from build123d import *

# Parameters (mm, degrees)
F1_DEPTH = 20


with BuildPart() as f1:
    # F0 (on Front) → F1 (new body)
    with BuildSketch(Plane.XZ):
        with BuildLine():
            ThreePointArc((6, -33), (4.404002, -27.946999), (0, -25))
            ThreePointArc((0, -25), (3.349365, -12.5), (0, 0))
            ThreePointArc((0, 0), (2.776172, 4.64825), (1.956342, 10))
            ThreePointArc((1.956342, 10), (-4.515013, 6.983663), (-6, 0))
            ThreePointArc((-6, 0), (-25.5, 3.94398), (-45, 0))
            ThreePointArc((-45, 0), (-47.052036, 6.711726), (-53.605872, 9.222772))
            ThreePointArc((-53.605872, 9.222772), (-53.826207, 4.173647), (-50.976141, 0))
            ThreePointArc((-50.976141, 0), (-54.905427, -13.454553), (-50.976141, -26.909107))
            ThreePointArc((-50.976141, -26.909107), (-54.301232, -29.687561), (-55.689886, -33.792153))
            ThreePointArc((-55.689886, -33.792153), (-49.556723, -34.118029), (-45, -30))
            ThreePointArc((-45, -30), (-25.5, -33.215544), (-6, -30))
            ThreePointArc((-6, -30), (-0.709551, -34.338204), (6, -33))
        make_face()
    extrude(amount=F1_DEPTH)


solid = f1.part
Geometry: final body of the model. Coordinates: model frame, mm. Give positions to 0.01 mm unless a question says otherwise; leave off trailing zeros. Loops run counter-clockwise (first coordinate to the right, second up) from the corner with the lowest first, then second, coordinate; pieces in that order, holes last. Notation, with made-up numbers: M 32,56.25 L 49,56.25 A14 cw 49,72.25 Z; hole C 64,-17.5 d9. An arc over 180 degrees is marked long. Put each result on its own line as item: value. Start each with the question number.
1) Ray query, line 1 along Z through (x, y) = (1.5, -18.25); line 2 along Z through (x, y) = (-52, -7); line 3 along X through (y, z) = (-10.75, 7.5). Return the intervals inside material, ascending.
2) Cut plane D-D (z = -14). Output: boundary loops of the cut face in (x, y), then the cut area to 3 significant figures.
3) Cut plane C-C (x = -35). Output: boundary loops of the cut face in (y, z), then the cut area to 3 significant figures.
4) Contact query for flat-ended pins moving along their axis: pin 1 (6 mm diameter, centred on x = -11, y = -12.5, fed in from +Z); pin 2 (2 mm diameter, centred on y = -12, z = -17, fed in from -X); pin 3 (1.5 mm diameter, centred on y = -5.5, z = -12.5, fed in from -X); pin 4 (6 mm diameter, centred on x = -26, z = -24.5, fed in from +Y). Output: stop coordinate, or through.
5) Cut plane B-B (y = -5). Output: boundary loops of the cut face in (x, z) (3 decimals).
6) Cut plane A-A (z = 6). Output: boundary loops of the cut face in (x, y).
7) Pull-direction query (Z, two-part tool) for faces 1 (the cylindrical face through (-49.64, -9.86, -34.147)), 2 (the cylindrical face through (3.35, -9.86, -12.68)), 3 (the flat face through (-25, -20, -12)), 4 (the cylindrical face through (-53.846, -9.86, 4.243)); classes: pulls with the +Z half, pulls with the -Z half, needs draft (parallel to the pull), parting line crosses it, or undercut.
Verdict:
1. line 1: -34.57 to -25.55, -21.94 to -3.06, 1.63 to 10
1. line 2: -34.58 to -27.46, -25.15 to -1.76, 0.93 to 9.2
1. line 3: -54.05 to -47.9, -4.07 to 2.82
2. outline: M -54.9,-20 L 3.3,-20 L 3.3,0 L -54.9,0 Z
2. area: 1,160 mm2
3. outline: M -20,-32.47 L 0,-32.47 L 0,3.04 L -20,3.04 Z
3. area: 710 mm2
4. pin 1: z = 2.61
4. pin 2: x = -54.78
4. pin 3: x = -54.9
4. pin 4: y = 0
5. outline: M -55.69,-33.792 A8 ccw -45,-30 A60.735 ccw -6,-30 A8 ccw 6,-33 A8 ccw 0,-25 A25 ccw 0,0 A8 ccw 1.956,10 A8 ccw -6,0 A50.178 ccw -45,0 A8 ccw -53.606,9.223 A8 ccw -50.976,0 A25 ccw -50.976,-26.909 A8 ccw Z
6. outline: M -54.12,-20 L -46.46,-20 L -46.46,0 L -54.12,0 Z; M -5.18,-20 L 2.92,-20 L 2.92,0 L -5.18,0 Z
7. face 1: pulls with the -Z half
7. face 2: undercut
7. face 3: needs draft
7. face 4: undercut
